```python
from build123d import *

# Parameters (mm, degrees)
F1_DEPTH = 25.4
F2_W     = 56.788672138
F2_H     = 0.0079375762
F2_R     = 17.5097347042
F3_DEPTH = 20.6140112132
F4_DEPTH = 25.4


with BuildPart() as f1:
    # F0 (on Top) → F1 (new body)
    with BuildSketch(Plane.XY):
        with BuildLine():
            Line((-45.808903873, -35.8836464584), (45.808903873, -35.8836464584))
            Line((45.808903873, -35.8836464584), (45.808903873, -31.8233038162))
            ThreePointArc((45.808903873, -31.8233038162), (37.8827370611, -28.5401780251), (34.5996112699, -20.6140112132))
            Line((34.5996112699, -20.6140112132), (-34.5996112699, -20.6140112132))
            ThreePointArc((-34.5996112699, -20.6140112132), (-37.8827370611, -28.5401780251), (-45.808903873, -31.8233038162))
            Line((-45.808903873, -31.8233038162), (-45.808903873, -35.8836464584))
        make_face()
        with BuildLine():
            ThreePointArc((-65.6594336033, -20.6140112132), (-59.4935648199, -33.1360447052), (-45.808903873, -35.8836464584))
            Line((-45.808903873, -35.8836464584), (-45.808903873, -31.8233038162))
            ThreePointArc((-45.808903873, -31.8233038162), (-53.7350706849, -28.5401780251), (-57.018196476, -20.6140112132))
            Line((-57.018196476, -20.6140112132), (-65.6594336033, -20.6140112132))
        make_face()
        with BuildLine():
            ThreePointArc((45.808903873, -35.8836464584), (58.3309373649, -31.6246287158), (65.6594336033, -20.6140112132))
            Line((65.6594336033, -20.6140112132), (57.018196476, -20.6140112132))
            ThreePointArc((57.018196476, -20.6140112132), (53.7350706849, -28.5401780251), (45.808903873, -31.8233038162))
            Line((45.808903873, -31.8233038162), (45.808903873, -35.8836464584))
        make_face()
        with BuildLine():
            Line((57.018196476, -20.6140112132), (65.6594336033, -20.6140112132))
            Line((65.6594336033, -20.6140112132), (65.6594336033, 20.6140112132))
            Line((65.6594336033, 20.6140112132), (-65.6594336033, 20.6140112132))
            Line((-65.6594336033, 20.6140112132), (-65.6594336033, -20.6140112132))
            Line((-65.6594336033, -20.6140112132), (-57.018196476, -20.6140112132))
            ThreePointArc((-57.018196476, -20.6140112132), (-45.808903873, -9.4047186102), (-34.5996112699, -20.6140112132))
            Line((-34.5996112699, -20.6140112132), (34.5996112699, -20.6140112132))
            ThreePointArc((34.5996112699, -20.6140112132), (45.808903873, -9.4047186102), (57.018196476, -20.6140112132))
        make_face()
    extrude(amount=F1_DEPTH)

    # F2 (on Front) → F3 (join, through all)
    with BuildSketch(Plane.XZ):
        with Locations((0, 25.3960312119)):
            Rectangle(F2_W, F2_H)
        with BuildLine():
            ThreePointArc((65.6594336033, 25.4), (39.3090304352, 36.3146943662), (28.394336069, 62.6650975343))
            Line((28.394336069, 62.6650975343), (28.394336069, 25.4))
            Line((28.394336069, 25.4), (45.808903873, 25.4))
            Line((45.808903873, 25.4), (65.6594336033, 25.4))
        make_face()
        with BuildLine():
            ThreePointArc((28.394336069, 115.8985176562), (0, 93.4414670745), (-28.394336069, 115.8985176562))
            Line((-28.394336069, 115.8985176562), (-28.394336069, 62.6650975343))
            Line((-28.394336069, 62.6650975343), (-28.394336069, 25.4))
            Line((-28.394336069, 25.4), (28.394336069, 25.4))
            Line((28.394336069, 25.4), (28.394336069, 62.6650975343))
            Line((28.394336069, 62.6650975343), (28.394336069, 115.8985176562))
        make_face()
        with BuildLine():
            Line((-28.394336069, 25.4), (-28.394336069, 62.6650975343))
            ThreePointArc((-28.394336069, 62.6650975343), (-39.3090304352, 36.3146943662), (-65.6594336033, 25.4))
            Line((-65.6594336033, 25.4), (-45.808903873, 25.4))
            Line((-45.808903873, 25.4), (-28.394336069, 25.4))
        make_face()
        with BuildLine():
            ThreePointArc((28.394336069, 115.8985176562), (28.9823181644, 119.2367591717), (29.179197795, 122.6206648695))
            ThreePointArc((29.179197795, 122.6206648695), (-3.3839056978, 151.6029830339), (-28.394336069, 115.8985176562))
            ThreePointArc((-28.394336069, 115.8985176562), (0, 93.4414670745), (28.394336069, 115.8985176562))
        make_face()
        with Locations((0, 122.6206648695)):
            Circle(F2_R, mode=Mode.SUBTRACT)
    extrude(amount=-F3_DEPTH)

    # F2 (on Front) → F4 (join)
    with BuildSketch(Plane.XZ):
        with BuildLine():
            ThreePointArc((28.394336069, 115.8985176562), (28.9823181644, 119.2367591717), (29.179197795, 122.6206648695))
            ThreePointArc((29.179197795, 122.6206648695), (-3.3839056978, 151.6029830339), (-28.394336069, 115.8985176562))
            ThreePointArc((-28.394336069, 115.8985176562), (0, 93.4414670745), (28.394336069, 115.8985176562))
        make_face()
        with Locations((0, 122.6206648695)):
            Circle(F2_R, mode=Mode.SUBTRACT)
    extrude(amount=F4_DEPTH)


solid = f1.part
```
Geometry check sheet. Reference: the model listing, model coordinates, mm. A direction names the side the tool comes from. Round coordinates to 2 decimals unless told otherwise and drop trailing zeros. Order: outer loops, then holes, each group sorted by start corner. A loop starts at its lowest first (then second) coordinate and runs counter-clockwise, first axis right, second up. Notation, with made-up numbers: (-17, -34) - (-9, -34) arc R11 ccw to (-9, -28) - close; hole circle Ø5 at (-8.5, 0.25). An arc over 180 degrees is marked (long way). Use a Markdown table: item, result. Add a question column.
1) Section check A-A (x = 0). Record the cut outline in (y, z), then the cut area to 3 significant figures.
2) Section check D-D (y = -5.5). Record the cut outline in (x, z), then the cut area to 3 significant figures.
3) Thickness scan on line 1 along Z through (x, y) = (0, -3); line 2 along X through (y, z) = (14.5, 123.5); line 3 along Y through (x, z) = (-7, 38). Record the ranges inside material, lowest first.
4) Gauge pin test, flat ends, axial feed: P1, Ø3, axis at y = -26, z = 109, coming from the +X side; P2, Ø22.5, axis at y = 8.5, z = 100, coming from the +X side; P3, Ø8, axis at x = 14.5, z = 34, coming from the -Y side. Record the tip position at first contact, or that the pin passes through.
5) Section check C-C (y = 16). Record the cut outline in (x, z).
6) Mould release check, pull along Z, two halves, no side actions. Record for faces 5 (the flat face through (1, 20.614, 58)), 6 (the flat face through (-1, -7, 0)), 7 (the cylindrical face through (2.97, -7.18, 151.65)), 8 (the flat face through (-1, 0, 61)): released by +Z, released by -Z, zero draft, split by the parting line, or undercut.
7) Set-up check for faces 1 (the flat face through (-1, -18, 25.4)), 2 (the flat face through (13, -25.4, 110)), 3 (the flat face through (-1, -35.884, 13)), 4 (the flat face through (28.394, 10, 89)): record each of +Z, -Z, +X, -X, +Y, -Y from which the full face is reachable in a straight line by a thin tool's end or side.
8) Section check B-B (y = -14). Record the cut outline in (x, z), then the cut area to 3 significant figures.
Established:
| question | item | result |
|---|---|---|
| 1 | outline | (-35.88, 0) - (20.61, 0) - (20.61, 105.11) - (-25.4, 105.11) - (-25.4, 93.44) - (0, 93.44) - (0, 25.4) - (-35.88, 25.4) - close; (-25.4, 140.13) - (20.61, 140.13) - (20.61, 151.8) - (-25.4, 151.8) - close |
| 1 | area | 3,910 mm2 |
| 2 | outline | (-65.66, 0) - (65.66, 0) - (65.66, 25.4) - (-65.66, 25.4) - close; circle Ø58.36 at (0, 122.62); hole circle Ø35.02 at (0, 122.62) |
| 2 | area | 5,050 mm2 |
| 3 | line 1 | 0 to 25.4, 93.44 to 105.11, 140.13 to 151.8 |
| 3 | line 2 | -29.17 to -17.49, 17.49 to 29.17 |
| 3 | line 3 | 0 to 20.61 |
| 4 | P1 | x = 26.49 |
| 4 | P2 | x = 28.39 |
| 4 | P3 | y = 0 |
| 5 | outline | (-65.66, 0) - (65.66, 0) - (65.66, 25.4) arc R37.27 cw to (28.39, 62.67) - (28.39, 115.9) arc R29.18 ccw (long way) to (-28.39, 115.9) - (-28.39, 62.67) arc R37.27 cw to (-65.66, 25.4) - close; hole circle Ø35.02 at (0, 122.62) |
| 6 | face 5 | zero draft |
| 6 | face 6 | released by -Z |
| 6 | face 7 | undercut |
| 6 | face 8 | undercut |
| 7 | face 1 | +X, -X, -Y |
| 7 | face 2 | +Z, +X, -X, -Y |
| 7 | face 3 | +Z, -Z, +X, -Y |
| 7 | face 4 | +X, +Y, -Y |
| 8 | outline | (-65.66, 0) - (-54.86, 0) - (-54.86, 25.4) - (-65.66, 25.4) - close; (-36.76, 0) - (36.76, 0) - (36.76, 25.4) - (-36.76, 25.4) - close; circle Ø58.36 at (0, 122.62); (54.86, 0) - (65.66, 0) - (65.66, 25.4) - (54.86, 25.4) - close; hole circle Ø35.02 at (0, 122.62) |
| 8 | area | 4,130 mm2 |
